from build123d import *

# Parameters (mm, degrees)
SKETCH1_R      = 0.5
SKETCH1_R_2    = 0.25
EXTRUDE1_DEPTH = 0.5


with BuildPart() as part:
    # Sketch1 → Extrude1 (new body)
    with BuildSketch(Plane(origin=(0, 0, 0), x_dir=(1, 0, 0), z_dir=(0, 1, 0))):
        with BuildLine():
            ThreePointArc((8.478240258, -4.538519193), (9, 0), (8.478240258, 4.538519193))
            ThreePointArc((8.478240258, 4.538519193), (7.071067812, 7.071067812), (4.538519193, 8.478240258))
            ThreePointArc((4.538519193, 8.478240258), (0, 9), (-4.538519193, 8.478240258))
            ThreePointArc((-4.538519193, 8.478240258), (-7.071067812, 7.071067812), (-8.478240258, 4.538519193))
            ThreePointArc((-8.478240258, 4.538519193), (-9, 0), (-8.478240258, -4.538519193))
            ThreePointArc((-8.478240258, -4.538519193), (-7.071067812, -7.071067812), (-4.538519193, -8.478240258))
            ThreePointArc((-4.538519193, -8.478240258), (0, -9), (4.538519193, -8.478240258))
            ThreePointArc((4.538519193, -8.478240258), (7.071067812, -7.071067812), (8.478240258, -4.538519193))
        make_face()
        with Locations((4, 4.5)):
            Circle(SKETCH1_R, mode=Mode.SUBTRACT)
        with Locations((-4, 4.5)):
            Circle(SKETCH1_R, mode=Mode.SUBTRACT)
        with Locations((4, -4.5)):
            Circle(SKETCH1_R, mode=Mode.SUBTRACT)
        with Locations((-4, -4.5)):
            Circle(SKETCH1_R, mode=Mode.SUBTRACT)
        with Locations((0, 6)):
            Circle(SKETCH1_R_2, mode=Mode.SUBTRACT)
        with Locations((0, -6)):
            Circle(SKETCH1_R_2, mode=Mode.SUBTRACT)
    extrude(amount=EXTRUDE1_DEPTH)


solid = part.part
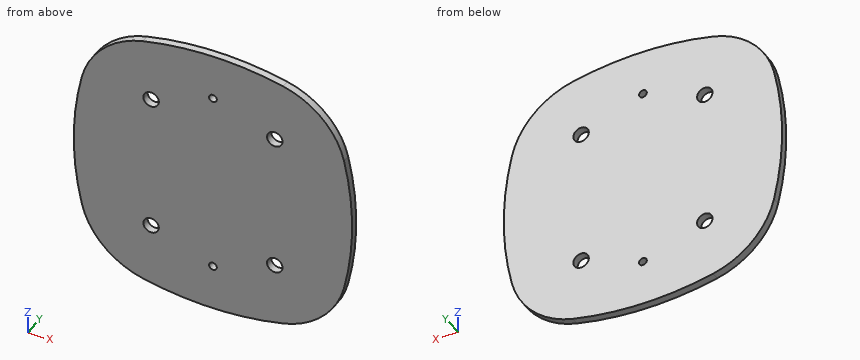
Can you work these out from the model? Positions are in its coordinate system, mm. Coordinates: 2 decimals unless noted, no trailing zeros. Loops run counter-clockwise (first coordinate to the right, second up) from the corner with the lowest first, then second, coordinate; pieces in that order, holes last. Notation, with made-up numbers: (83.25, 42.5) - (135.25, 42.5) arc R17 ccw to (135.25, 48.5) - close; hole circle Ø4 at (83.25, 64.5). An arc over 180 degrees is marked (long way). Answer as a JSON object with one key per item and string values. Group by question number.
Item 1: If we section it at B-B (y = 0.3): List the corners of the cut face in (x, z) for me.
Item 2: If we section it at A-A (x = 0): List the corners of the cut face in (y, z) for me.
Item 3: If we section it at C-C (z = 4.25): List the corners of the cut face in (x, y) for me, plus the area to 3 significant figures.
Item 4: If I drill on L1, parallel to Z at x = 0, y = 0.1; L2, parallel to Z at x = -4, y = 0.3; L3, parallel to X at y = 0.2, z = 4.5, over which ranges is the centre line in solid material (lowest first)? Write a range as from..to.
Item 5: If we section it at D-D (z = -6): List the corners of the cut face in (x, y) for me, plus the area to 3 significant figures.
Returned:
{
 "1": {"outline": "(-8.48, -4.54) arc R5.27 ccw to (-4.54, -8.48) arc R20 ccw to (4.54, -8.48) arc R5.27 ccw to (8.48, -4.54) arc R20 ccw to (8.48, 4.54) arc R5.27 ccw to (4.54, 8.48) arc R20 ccw to (-4.54, 8.48) arc R5.27 ccw to (-8.48, 4.54) arc R20 ccw to start; hole circle Ø1 at (-4, -4.5); hole circle Ø1 at (-4, 4.5); hole circle Ø0.5 at (0, -6); hole circle Ø0.5 at (0, 6); hole circle Ø1 at (4, -4.5); hole circle Ø1 at (4, 4.5)"},
 "2": {"outline": "(0, -9) - (0.5, -9) - (0.5, -6.25) - (0, -6.25) - close; (0, -5.75) - (0.5, -5.75) - (0.5, 5.75) - (0, 5.75) - close; (0, 6.25) - (0.5, 6.25) - (0.5, 9) - (0, 9) - close"},
 "3": {"outline": "(-8.54, 0) - (-4.43, 0) - (-4.43, 0.5) - (-8.54, 0.5) - close; (-3.57, 0) - (3.57, 0) - (3.57, 0.5) - (-3.57, 0.5) - close; (4.43, 0) - (8.54, 0) - (8.54, 0.5) - (4.43, 0.5) - close", "area": "7.68 mm²"},
 "4": {"L1": "z = -9..-6.25, -5.75..5.75, 6.25..9", "L2": "z = -8.6..-5, -4..4, 5..8.6", "L3": "x = -8.49..-4.5, -3.5..3.5, 4.5..8.49"},
 "5": {"outline": "(-7.9, 0) - (-0.25, 0) - (-0.25, 0.5) - (-7.9, 0.5) - close; (0.25, 0) - (7.9, 0) - (7.9, 0.5) - (0.25, 0.5) - close", "area": "7.65 mm²"}
}
